Can you work these out from the model? Positions are in its coordinate system, mm. A direction names the side the tool comes from. Coordinates: 2 decimals unless noted, no trailing zeros. Loops run counter-clockwise (first coordinate to the right, second up) from the corner with the lowest first, then second, coordinate; pieces in that order, holes last. Notation, with made-up numbers: M 31.5,79 L 57.5,79 A29 ccw 57.5,107 Z; hole C -20.5,20 d1. An arc over 180 degrees is marked long. Answer as a JSON object with one key per item and string values. Group by question number.
Item 1: I'm going to push flat-ended pins straight in: pin 1 Ø2 at (x, z) = (-53, -14) entering from +Y; pin 2 Ø18 at (y, z) = (68, -9) entering from -X; pin 3 Ø13 at (x, z) = (38.72, 0) entering from +Y; pin 4 Ø8 at (x, z) = (28, 15) entering from -Y. Where does each tip first touch, or does it pass through?
Item 2: Suppose I cut it at B-B (z = 0). Write out the boundary of the cut face in (x, y), then the cut area to 3 significant figures.
Item 3: Which directions (+Z, -Z, +X, -X, +Y, -Y) give clear straight access to the entire face, cutting with the end or side of a thin tool? Please do faces 4 (the flat face through (39, 84, 10)), 5 (the cylindrical face through (-36.129, 17.042, 4.868)), 6 (the flat face through (-0.98, 6.9, -14.71)).
Item 4: Suppose I cut it at A-A (y = 75.5). Write out the boundary of the cut face in (x, z), then the cut area to 3 significant figures.
Item 5: Suppose I cut it at C-C (z = -22). Write out the boundary of the cut face in (x, y).
Item 6: We'd pull the mould along X, two halves only. Please class faces 1 (the flat face through (70, 43, 0)), 2 (the cylindrical face through (4.589, 36.129, 4.868)), 3 (the flat face through (-31, 50, 0)): +X half, -X half, draft (parallel to the pull), parting line (faces both ways), or undercut.
Item 7: Suppose I cut it at D-D (x = 57). Write out the boundary of the cut face in (y, z).
Item 8: If I drill on line 1 (Y direction, x = 18, z = 0); line 2 (Y direction, x = -3, z = 0); line 3 (X direction, y = 52.75, z = 0), over which ranges is the centre line in solid material (lowest first)?
```python
from build123d import *

# Parameters (mm, degrees)
BOSS_EXTRUDE1_DEPTH = 27.5
CUT_EXTRUDE1_DEPTH  = 169.689804078
CUT_EXTRUDE2_DEPTH  = 63
SKETCH7_R           = 8
FILLET1_R           = 2
FILLET2_R           = 2


with BuildPart() as part:
    # Sketch1 → Boss-Extrude1 (new, symmetric)
    with BuildSketch(Plane.XY):
        Polygon((-70, 0), (70, 0), (70, 90), (7, 90), (7, 50), (-70, 50), align=None)
    extrude(amount=BOSS_EXTRUDE1_DEPTH, both=True)

    # Sketch3 → Cut-Extrude1 (cut, through all)
    with BuildSketch(Plane.ZY.offset(70)):
        Polygon((-12, 0), (-17.5, 14), (17.5, 14), (12, 0), align=None)
    extrude(amount=-CUT_EXTRUDE1_DEPTH, mode=Mode.SUBTRACT)

    # Sketch5 → Cut-Extrude2 (cut)
    with BuildSketch(Plane(origin=(70, 0, 0), x_dir=(0, 0, -1), z_dir=(1, 0, 0))):
        Polygon((-10, 90), (-10, 78), (-20, 78), (-20, 63), (20, 63), (20, 78), (10, 78), (10, 90), align=None)
    extrude(amount=-CUT_EXTRUDE2_DEPTH, mode=Mode.SUBTRACT)

    # Cut-Sweep2: sweep along a path in Sketch6
    with BuildLine(Plane.XY) as cut_sweep2_path:
        Line((-30, 14), (-30, 20))
        ThreePointArc((-30, 20), (-27.071067812, 27.071067812), (-20, 30))
        Line((-20, 30), (28.5, 30))
        ThreePointArc((28.5, 30), (35.571067812, 32.928932188), (38.5, 40))
        Line((38.5, 40), (38.5, 63))
    # Sketch7 → Cut-Sweep2 (sweep, cut)
    with BuildSketch(Plane(origin=(38.5, 63, 0), x_dir=(1, 0, 0), z_dir=(0, 1, 0))):
        with Locations((0.219622083, 0)):
            Circle(SKETCH7_R)
    sweep(path=cut_sweep2_path.line, mode=Mode.SUBTRACT)

    # Fillet1
    fillet1_edges = [part.edges().sort_by_distance(p)[0] for p in [
        (-70, 50, 0),
        (7, 50, 0),
        (7, 90, 18.75),
        (7, 90, -18.75),
    ]]
    fillet(fillet1_edges, radius=FILLET1_R)

    # Fillet2
    fillet2_edges = [part.edges().sort_by_distance(p)[0] for p in [
        (70, 90, 18.75),
        (70, 90, -18.75),
    ]]
    fillet(fillet2_edges, radius=FILLET2_R)


solid = part.part
```
From the geometry:
{
 "1": {"pin 1": "y = 50", "pin 2": "x = 7", "pin 3": "y = 32.76", "pin 4": "y = 0"},
 "2": {"outline": "M -70,14 L -37.78,14 L -37.78,20 A17.78 cw -20,37.78 L 28.5,37.78 A2.22 ccw 30.72,40 L 30.72,63 L 7,63 L 7,52 A2 cw 5,50 L -68,50 A2 ccw -70,48 Z; M -21.78,14 L 70,14 L 70,63 L 46.72,63 L 46.72,40 A18.22 cw 28.5,21.78 L -20,21.78 A1.78 ccw -21.78,20 Z", "area": "4,120 mm2"},
 "3": {"face 4": "+X, -X, +Y", "face 5": "-Y", "face 6": "+X, -X"},
 "4": {"outline": "M 7,-27.5 L 70,-27.5 L 70,-20 L 7,-20 Z; M 7,20 L 70,20 L 70,27.5 L 7,27.5 Z", "area": "945 mm2"},
 "5": {"outline": "M -70,0 L 70,0 L 70,88 A2 ccw 68,90 L 9,90 A2 ccw 7,88 L 7,52 A2 cw 5,50 L -68,50 A2 ccw -70,48 Z"},
 "6": {"face 1": "+X half", "face 2": "undercut", "face 3": "draft"},
 "7": {"outline": "M 0,-27.5 L 90,-27.5 L 90,-10 L 78,-10 L 78,-20 L 63,-20 L 63,20 L 78,20 L 78,10 L 90,10 L 90,27.5 L 0,27.5 L 0,12 L 14,17.5 L 14,-17.5 L 0,-12 Z"},
 "8": {"line 1": "14 to 21.78, 37.78 to 63", "line 2": "14 to 21.78, 37.78 to 50", "line 3": "7 to 30.72, 46.72 to 70"}
}
